Can you work these out from the model? Positions are in its coordinate system, mm. Face numbers are marked on the shaded views. A direction names the side the tool comes from. Coordinates: 2 decimals unless noted, no trailing zeros. Order: outer loops, then holes, each group sorted by start corner. A loop starts at its lowest first (then second) coordinate and runs counter-clockwise, first axis right, second up. Notation, with made-up numbers: (-21, -1.5) -> (32, -1.5) arc R11 cw to (32, 7.5) -> close; hole circle Ø1 at (24.25, 11). An arc over 180 degrees is marked (long way). Answer as CSV lines item,"result".
from build123d import *

# Parameters (mm, degrees)
SKETCH_1_R      = 1
EXTRUDE_1_DEPTH = 8
FILLET_3_R      = 0.5


with BuildPart() as part:
    # 草圖1 → 填料-伸長1 (new body)
    with BuildSketch(Plane(origin=(0, 0, 0), x_dir=(1, 0, 0), z_dir=(0, 1, 0))):
        with BuildLine():
            Line((0, 0), (0, 12.2))
            Line((0, 12.2), (-22.5, 12.2))
            Line((-22.5, 12.2), (-22.5, 0))
            Line((-22.5, 0), (-27.124303732, 0))
            ThreePointArc((-27.124303732, 0), (-31.398520886, 0.462060812), (-35.475243216, 1.826893228))
            Line((-35.475243216, 1.826893228), (-55.835093948, 11.182689323))
            ThreePointArc((-55.835093948, 11.182689323), (-56.953793919, 13.427421715), (-55, 15))
            Line((-55, 15), (5, 15))
            ThreePointArc((5, 15), (12.5, 7.5), (5, 0))
            Line((5, 0), (0, 0))
        make_face()
        with Locations(Location((-25, 6.1, 0), (0, 0, 270))):
            Circle(SKETCH_1_R, mode=Mode.SUBTRACT)
        with Locations(Location((2.5, 6.1, 0), (0, 0, 270))):
            Circle(SKETCH_1_R, mode=Mode.SUBTRACT)
    extrude(amount=EXTRUDE_1_DEPTH)

    # 圓角3
    fillet_3_edges = [part.edges().sort_by_distance(p)[0] for p in [
        (-25, 8, -15),
        (-24.812151866, 0, 0),
        (-31.398520886, 0, -0.462060812),
        (-45.655168582, 0, -6.504791275),
        (-56.953793919, 0, -13.427421715),
        (-25, 0, -15),
        (12.5, 0, -7.5),
        (2.5, 0, 0),
        (-56.953793919, 8, -13.427421715),
        (-45.655168582, 8, -6.504791275),
        (0, 4, 0),
        (-22.5, 4, 0),
        (-31.398520886, 8, -0.462060812),
        (-24.812151866, 8, 0),
        (2.5, 8, 0),
        (12.5, 8, -7.5),
    ]]
    fillet(fillet_3_edges, radius=FILLET_3_R)


solid = part.part
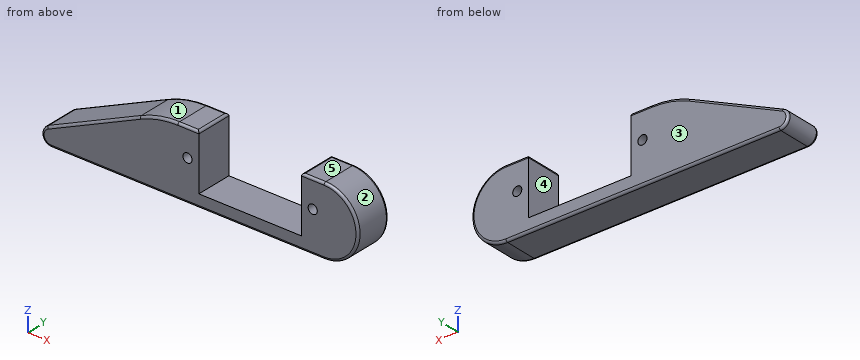
Q1. Imagine slicing it at C-C (x = -20). List the corners of the cut face in (y, z) for me, and give its area (3 significant figures).
Solution:
outline,"(0, -14.5) arc R0.5 ccw to (0.5, -15) -> (7.5, -15) arc R0.5 ccw to (8, -14.5) -> (8, -12.2) -> (0, -12.2) -> close"
area,"22.3 mm2"
Q2. If I drill on line 1 (X direction, y = 3.25, z = -6.1); line 2 (Z direction, x = -8, y = 3); line 3 (X direction, y = 5, z = -3.5), over which ranges is the centre line in solid material (lowest first)?
Solution:
line 1,"-44.77 to -26, -24 to -22.5, 0 to 1.5, 3.5 to 12.37"
line 2,"-15 to -12.2"
line 3,"-39.12 to -22.5, 0 to 11.34"
Q3. Which directions (+Z, -Z, +X, -X, +Y, -Y) give clear straight access to the entire face, cutting with the end or side of a thin tool? Please do the marked faces 4 and 5.
Solution:
face 4,"+Z, +Y, -Y"
face 5,"+Z, +X, -X, +Y, -Y"
Q4. Imagine slicing it at A-A (x = 2.5). List the corners of the cut face in (y, z) for me, and give its area (3 significant figures).
Solution:
outline,"(0, -14.5) arc R0.5 ccw to (0.5, -15) -> (7.5, -15) arc R0.5 ccw to (8, -14.5) -> (8, -7.1) -> (0, -7.1) -> close; (0, -5.1) -> (8, -5.1) -> (8, -0.5) arc R0.5 ccw to (7.5, 0) -> (0.5, 0) arc R0.5 ccw to (0, -0.5) -> close"
area,"104 mm2"
Q5. Imagine slicing it at B-B (y = 5.25). List the corners of the cut face in (x, z) for me.
Solution:
outline,"(-55.84, -11.18) arc R2 ccw to (-55, -15) -> (5, -15) arc R7.5 ccw to (5, 0) -> (0.5, 0) arc R0.5 ccw to (0, -0.5) -> (0, -12.2) -> (-22.5, -12.2) -> (-22.5, -0.5) arc R0.5 ccw to (-23, 0) -> (-27.12, 0) arc R20 ccw to (-35.48, -1.83) -> close; hole circle Ø2 at (-25, -6.1); hole circle Ø2 at (2.5, -6.1)"
Q6. Imagine slicing it at D-D (z = -6.25). Give the number of separate pieces and of enclosed holes in the cut face, and give its area (3 significant figures).
Solution:
separate pieces,"4"
enclosed holes,"0"
area,"248 mm2"
Q7. For P1, Ø2.5, axis at y = 6, z = -4, coming from the -X side; P2, Ø3, axis at y = 5, z = -12.5, coming from the +X side; P3, Ø4, axis at x = -14.5, y = 4, coming from the +Z side, each with a flat end and sliding along its axis, tell me the tip position at first contact or that it passes through.
Solution:
P1,"x = -42.92"
P2,"x = 11.63"
P3,"z = -12.2"
Q8. We'd pull the mould along Z, two halves only. Please class the marked faces 1, 2 and 3: pulls with the +Z half, pulls with the -Z half, needs draft (parallel to the pull), parting line crosses it, or undercut.
Solution:
face 1,"pulls with the +Z half"
face 2,"parting line crosses it"
face 3,"needs draft"
